Verification items for this drawing (mm, ordinates from the low corner). A direction names the side the tool comes from. Round coordinates to 2 decimals unless told otherwise and drop trailing zeros. Loops run counter-clockwise (first coordinate to the right, second up) from the corner with the lowest first, then second, coordinate; pieces in that order, holes last. Notation, with made-up numbers: M 73,13 L 105,13 A25 ccw 105,41 Z; hole C 37.25,14 d7. An arc over 180 degrees is marked long. Use one line per item in the form item = value. Start each with the question number.
1. Go/stop test with flat-tipped pins: pin 1 (3 mm diameter, centred on x = 16, z = 13, fed in from -Y); pin 2 (4 mm diameter, centred on x = 14.5, y = 16, fed in from +Z); pin 3 (2 mm diameter, centred on x = 10.5, y = 28.5, fed in from -Z). Record where each tip stops, or that it passes through.
2. Cross-section at C-C (y = 25). Record the boundary of the cut face in (x, z), then the cut area to 3 significant figures.
3. Material ranges on line 1 (X direction, y = 14.75, z = 16.5); line 2 (Y direction, x = 14.5, z = 18.25); line 3 (Z direction, x = 5.5, y = 27), recorded low to high.
4. Cross-section at B-B (z = 5). Record the boundary of the cut face in (x, y).
5. Cross-section at D-D (z = 15). Record the boundary of the cut face in (x, y), then the cut area to 3 significant figures.
6. Cross-section at A-A (x = 10). State how many separate pieces and enclosed holes the cut face has, then the cut area to 3 significant figures.
7. Set-up check for the marked faces 5, 6, 7, 8 and 9: record each of +Z, -Z, +X, -X, +Y, -Y from which the full face is reachable in a straight line by a thin tool's end or side.
8. Draft check along X on the marked faces 1, 2, 3 and 4. Enter one of: pulls with the +X half, pulls with the -X half, needs draft (parallel to the pull), parting line crosses it, or undercut.
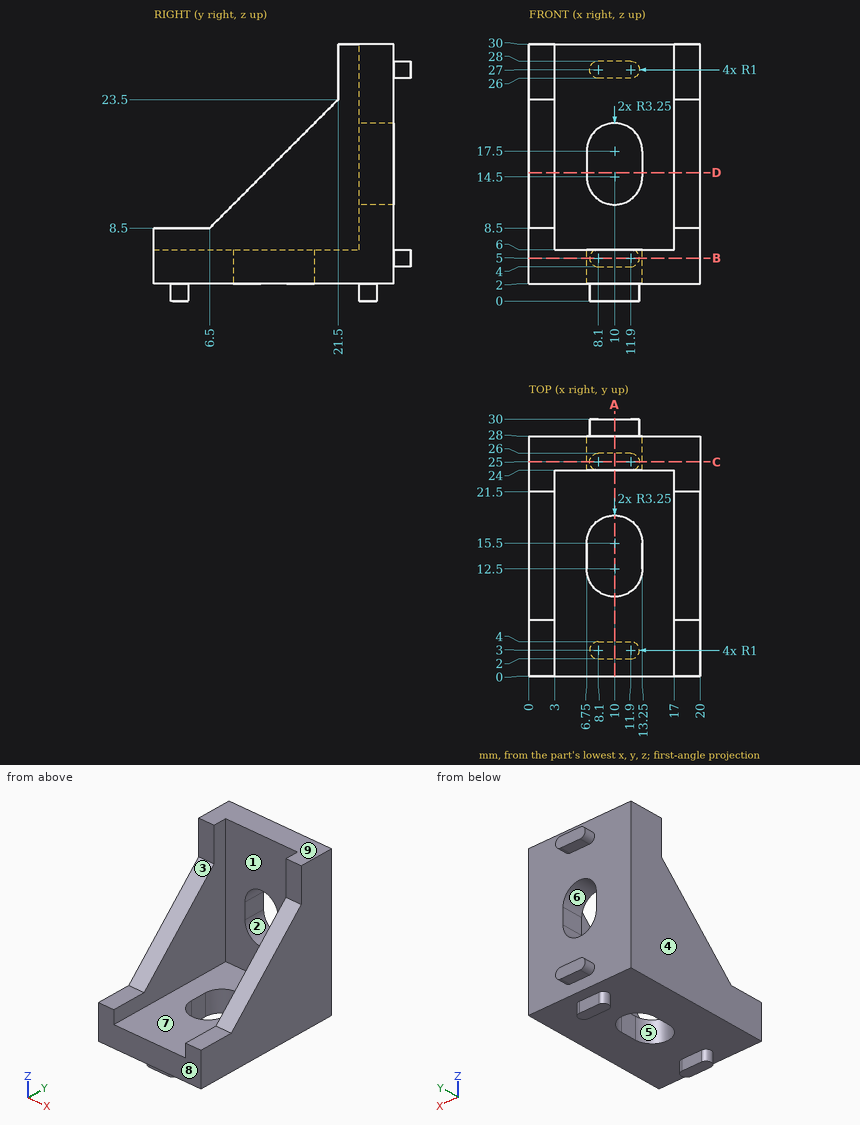
Reported:
q1.pin_1 = 9.88
q1.pin_2 = 6
q1.pin_3 = 2
q2.outline = M 0,2 L 7.1,2 L 7.1,0 L 12.9,0 L 12.9,2 L 20,2 L 20,30 L 0,30 Z; hole M 6.75,14.5 A3.25 ccw 13.25,14.5 L 13.25,17.5 A3.25 ccw 6.75,17.5 Z
q2.area = 519 mm²
q3.line_1 = 0 to 3, 17 to 20
q3.line_2 = 24 to 28
q3.line_3 = 2 to 30
q4.outline = M 0,0 L 20,0 L 20,28 L 12.9,28 L 12.9,30 L 7.1,30 L 7.1,28 L 0,28 Z; hole M 6.75,12.5 A3.25 ccw 13.25,12.5 L 13.25,15.5 A3.25 ccw 6.75,15.5 Z
q5.outline = M 0,13 L 3,13 L 3,24 L 6.75,24 L 6.75,28 L 0,28 Z; M 13.25,24 L 17,24 L 17,13 L 20,13 L 20,28 L 13.25,28 Z
q5.area = 120 mm²
q6.separate_pieces = 3
q6.enclosed_holes = 0
q6.area = 148 mm²
q7.face_5 = +Z, -Z
q7.face_6 = +Y, -Y
q7.face_7 = +Z, -Y
q7.face_8 = +Z, -Z, +X, -X, -Y
q7.face_9 = +Z, +X, -X, +Y, -Y
q8.face_1 = undercut
q8.face_2 = undercut
q8.face_3 = needs draft
q8.face_4 = pulls with the -X half
